Build history of the part. All positions in model axes, mm. Face numbers are marked on the shaded views. A direction names the side the tool comes from. Coordinates: 2 decimals unless noted, no trailing zeros. Order: outer loops, then holes, each group sorted by start corner. A loop starts at its lowest first (then second) coordinate and runs counter-clockwise, first axis right, second up. Notation, with made-up numbers: M 27.5,-34 L 69.5,-34 A17 ccw 69.5,-8 Z; hole C -3,31.25 d11. An arc over 180 degrees is marked long. Write item = value, one per line. Start each with the question number.
Q1. Band-saw the part on A-A on z = 0.15. Write the cut outline in (x, y) (3 decimals).
Q2. Pin check, flat tips, straight feed: P1, Ø1.6, axis at x = 0.5, y = 1, coming from the +Z side; P2, Ø2, axis at x = 4.5, y = 7, coming from the -Z side. Stop position of each tip, or through.
Q3. 3-axis set-ups, long thin cutter, end or side, ignore diameter. For the marked faces 1 and 2: which of +Z, -Z, +X, -X, +Y, -Y reach the whole face in a straight line?
Q4. Band-saw the part on B-B on x = 0. Write the cut outline in (y, z).
Q5. Band-saw the part on C-C on z = -2.5. Write the cut outline in (x, y), plus the area to 3 significant figures.
Q6. Pull direction X, two halves, no side cores. Call the marked faces 3, 4 and 5: released by +X, released by -X, zero draft, split by the parting line, or undercut.
Q7. Drill centre lines: probe 1 along Y at (x, z) = (0, -1.9); probe 2 along Z at (x, y) = (-2.75, 7); probe 3 along Z at (x, y) = (0.25, -2). Where is each one in solid material? Low to high.
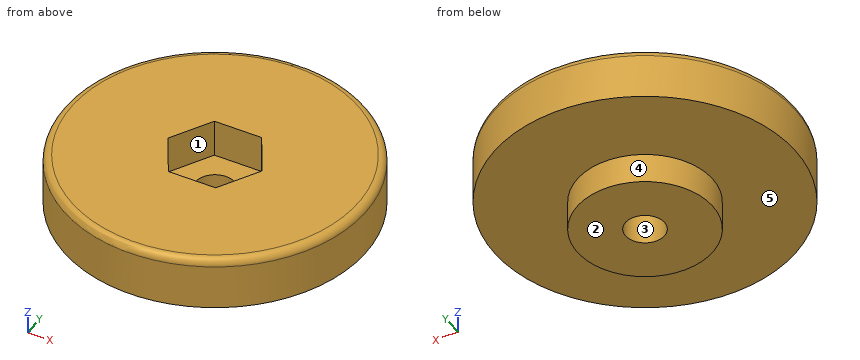
Autodesk Inventor part; units mm, degrees
ref_plane "РабПлоскость2" through (-7.5, 5, 1.5) normal (0, 0, 1) x (1, 0, 0)
ref_plane "YZ Plane" through (0, 0, 0) normal (1, 0, 0) x (0, 1, 0)
ref_plane "XZ Plane" through (0, 0, 0) normal (0, 1, 0) x (-1, 0, 0)
sketch "Эскиз1" plane through (0, 0, 0) normal (0, 1, 0) x (-1, 0, 0)
  line L0 (-10, 1.75) -> (10, 1.75)
  line L1 (10, 1.75) -> (10, -1.75)
  line L2 (10, -1.75) -> (-10, -1.75)
  line L3 (-10, -1.75) -> (-10, 1.75)
  line L4 (-10, 1.75) -> (10, -1.75) construction
  line L5 (10, 1.75) -> (-10, -1.75) construction
  line L6 (2.5, -1.75) -> (-2.5, -1.75)
  line L7 (-2.5, -1.75) -> (-2.5, -3.95)
  line L8 (-2.5, -3.95) -> (2.5, -3.95)
  line L9 (2.5, -3.95) -> (2.5, -1.75)
  line L10 (0, 1.75) -> (0, -1.75)
  point P0 (0, 0)
  dimension "d0" = 20
  dimension "d1" = 3.5
  dimension "d2" = 5
  dimension "d3" = 2.2
revolve "Вращение1" add sketch "Эскиз1" angle 360 about axis through (0, 0, 1.75) along (0, 0, -1) contours L0 L1 L2 L10
ref_plane "РабПлоскость2" through (-7.5, 5, 1.5) normal (0, 0, 1) x (1, 0, 0)
sketch "Эскиз4" plane through (0, 0, -1.75) normal (0, 0, -1) x (-1, 0, 0)
  circle A0 centre (0, 0) radius 1.3
  circle A1 centre (0, 0) radius 4.5
  point P0 (0, 0)
  dimension "d20" = 2.6
  dimension "d21" = 9
extrude "Выдавливание5" add sketch "Эскиз4" along normal blind 2
extrude "Выдавливание6" cut sketch "Эскиз4" against normal mid plane 12 contours A0
fillet "Сопряжение1" radius 0.5 1 edges at (10, 0, 1.75)
sketch "Эскиз5" plane through (0, 0, 1.75) normal (0, 0, 1) x (1, 0, 0)
  circle A0 centre (0, 0) radius 3.15 construction
  line L0 (0, 0) -> (1.575, 2.728) construction
  line L1 (0, 0) -> (-1.575, 2.728) construction
  line L2 (0, 0) -> (-3.15, 0) construction
  line L3 (0, 0) -> (-1.575, -2.728) construction
  line L4 (0, 0) -> (1.575, -2.728) construction
  line L5 (0, 0) -> (3.15, 0) construction
  line L6 (1.575, 2.728) -> (3.15, 0)
  line L7 (-1.575, 2.728) -> (1.575, 2.728)
  line L8 (-3.15, 0) -> (-1.575, 2.728)
  line L9 (-1.575, -2.728) -> (-3.15, 0)
  line L10 (1.575, -2.728) -> (-1.575, -2.728)
  line L11 (3.15, 0) -> (1.575, -2.728)
  point P0 (0, 0)
  point P1 (-1.575, -2.728)
  point P2 (3.15, 0)
  point P3 (1.575, 2.728)
  dimension "d29" = 6.3
  dimension "d32" = 360
  dimension "d36" = 360
extrude "Выдавливание7" cut sketch "Эскиз5" against normal blind 2.5
properties part number "kikcer_head_001"
Recorded:
q1.outline = C 0,0 d20; hole M -3.15,0 L -1.575,-2.728 L 1.575,-2.728 L 3.15,0 L 1.575,2.728 L -1.575,2.728 Z
q2.P1 = -0.75
q2.P2 = -1.75
q3.face_1 = +Z
q3.face_2 = -Z, +X, -X, +Y, -Y
q4.outline = M -10,-1.75 L -4.5,-1.75 L -4.5,-3.75 L -1.3,-3.75 L -1.3,-0.75 L -2.73,-0.75 L -2.73,1.75 L -9.5,1.75 A0.5 ccw -10,1.25 Z; M 1.3,-3.75 L 4.5,-3.75 L 4.5,-1.75 L 10,-1.75 L 10,1.25 A0.5 ccw 9.5,1.75 L 2.73,1.75 L 2.73,-0.75 L 1.3,-0.75 Z
q5.outline = C 0,0 d9; hole C 0,0 d2.6
q5.area = 58.3 mm2
q6.face_3 = undercut
q6.face_4 = split by the parting line
q6.face_5 = zero draft
q7.probe_1 = -4.5 to -1.3, 1.3 to 4.5
q7.probe_2 = -1.75 to 1.75
q7.probe_3 = -3.75 to -0.75
